Build history of the part. All positions in model axes, mm. Face numbers are marked on the shaded views. Give positions to 0.01 mm unless a question says otherwise; leave off trailing zeros. Write each loop counter-clockwise with the first axis right and the second up, starting at its lowest first coordinate (ties: lowest second). Pieces come first, ordered by that corner, then holes. Notation, with made-up numbers: M 26.25,68 L 58.25,68 A23 cw 58.25,93 Z; hole C 66.5,38 d7. An arc over 180 degrees is marked long. Return JSON: item names as keys, results as strings. Group by question number.
Q1. Band-saw the part on C-C, the plane y = 12. Give the cut face in (x, z).
Q2. Pull direction X, two halves, no side cores. Call the marked faces 1, 2, 3 and 4: +X half, -X half, draft (parallel to the pull), parting line (faces both ways), or undercut.
Q3. Flat gauge pins, fed straight in: pin 1 Ø2 at (x, z) = (-18, 7.5) entering from -Y; pin 2 Ø12 at (y, z) = (53.5, -16.5) entering from -X; pin 3 Ø8 at (x, z) = (-43.5, -45.5) entering from +Y; pin 4 Ø1.5 at (x, y) = (-17.5, 57) entering from +Z. Where does each tip first touch, or does it go through?
Q4. Band-saw the part on B-B, the plane z = 0. Give the cut face in (x, y).
Q5. Band-saw the part on A-A, the plane x = 0. Give the cut face in (y, z), then the cut area to 3 significant figures.
Q6. Wall check: probe 1 along Y at (x, z) = (3.5, -38); probe 2 along X at (y, z) = (69, 47.5); probe 3 along X at (y, z) = (10, 22.5). Give the ranges that are in metal, low to high.
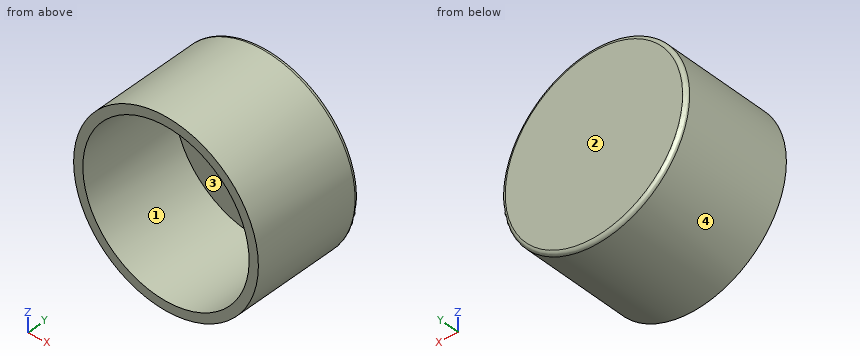
from build123d import *

# Parameters (mm, degrees)
SKETCH1_R           = 63.5
BOSS_EXTRUDE1_DEPTH = 76.2
SHELL1_T            = -6.35
FILLET1_R           = 2.54


with BuildPart() as part:
    # Sketch1 → Boss-Extrude1 (new body)
    with BuildSketch(Plane(origin=(0, 0, 0), x_dir=(1, 0, 0), z_dir=(0, 1, 0))):
        with Locations(Location((0, 0, 0), (0, 0, 90))):
            Circle(SKETCH1_R)
    extrude(amount=BOSS_EXTRUDE1_DEPTH)

    # Shell1
    shell1_openings = [part.faces().sort_by_distance(p)[0] for p in [
        (0, 0, 0),
    ]]
    offset(amount=SHELL1_T, openings=shell1_openings, kind=Kind.INTERSECTION)

    # Fillet1
    fillet1_edges = [part.edges().sort_by_distance(p)[0] for p in [
        (0, 76.2, 63.5),
    ]]
    fillet(fillet1_edges, radius=FILLET1_R)


solid = part.part
From the geometry:
{
 "1": {"outline": "C 0,0 d127; hole C 0,0 d114.3"},
 "2": {"face 1": "undercut", "face 2": "draft", "face 3": "undercut", "face 4": "parting line"},
 "3": {"pin 1": "stops at y = 69.85", "pin 2": "stops at x = -62.63", "pin 3": "stops at y = 76.2", "pin 4": "stops at z = 61.25"},
 "4": {"outline": "M -63.5,0 L -57.15,0 L -57.15,69.85 L 57.15,69.85 L 57.15,0 L 63.5,0 L 63.5,73.66 A2.54 ccw 60.96,76.2 L -60.96,76.2 A2.54 ccw -63.5,73.66 Z"},
 "5": {"outline": "M 0,-63.5 L 73.66,-63.5 A2.54 ccw 76.2,-60.96 L 76.2,60.96 A2.54 ccw 73.66,63.5 L 0,63.5 L 0,57.15 L 69.85,57.15 L 69.85,-57.15 L 0,-57.15 Z", "area": "1,690 mm^2"},
 "6": {"probe 1": "y = 69.85 to 76.2", "probe 2": "x = -42.14 to -31.78, 31.78 to 42.14", "probe 3": "x = -59.38 to -52.53, 52.53 to 59.38"}
}
